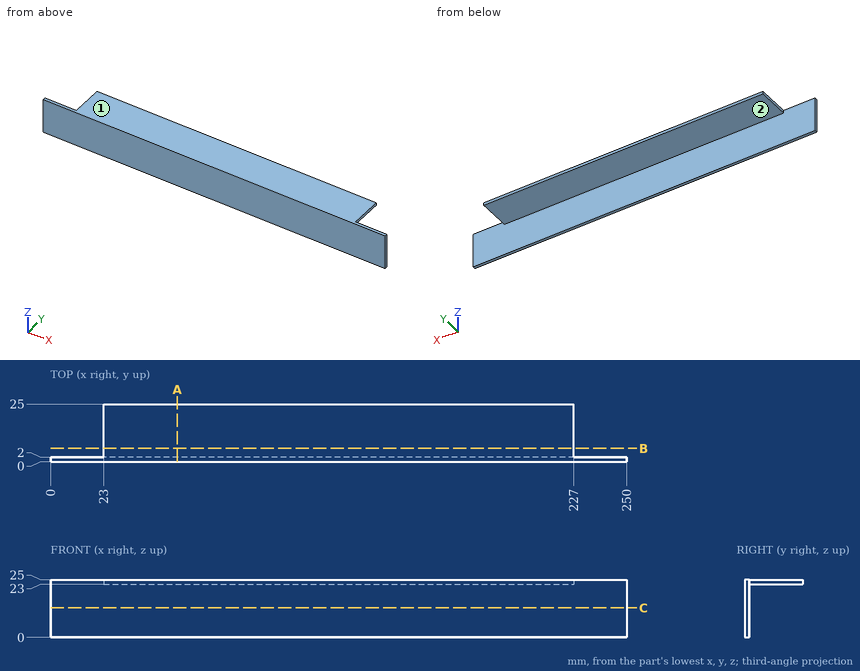
Input: dimensioned drawing with shaded views. Units: mm. Origin: part minimum x, y, z. A direction names the side the tool comes from. Coordinates: 2 decimals unless noted, no trailing zeros. Order: outer loops, then holes, each group sorted by start corner. A loop starts at its lowest first (then second) coordinate and runs counter-clockwise, first axis right, second up.
1. Ray query, line 1 along Y through (x, z) = (131.5, 4); line 2 along Z through (x, y) = (185, 15.5). Return the intervals inside material, ascending.
Checked values:
line 1: y = 0 to 2
line 2: z = 23 to 25
2. Cut plane C-C, the plane z = 12.75. Return loops of the section in (x, y).
Checked values:
outline: (0, 0) - (250, 0) - (250, 2) - (0, 2) - close
3. Access query for the marked faces 1 and 2. Directions: +Z, -Z, +X, -X, +Y, -Y. A direction counts if a zero-diameter tool reaches every point of the face in a straight line with its end or side. Return the directions, or none.
Checked values:
face 1: +Z, +X, -X, +Y, -Y
face 2: -Z, +X, -X, +Y
4. Contact query for flat-ended pins moving along their axis: P1, Ø12, axis at x = 221.5, y = 20.5, coming from the -Z side; P2, Ø12, axis at y = 12, z = 19, coming from the -X side; P3, Ø0.6, axis at y = 11.5, z = 24, coming from the +X side. Output: stop coordinate, or through.
Checked values:
P1: stops at z = 23
P2: stops at x = 23
P3: stops at x = 227
5. Cut plane A-A, the plane x = 55. Return loops of the section in (y, z).
Checked values:
outline: (0, 0) - (2, 0) - (2, 23) - (25, 23) - (25, 25) - (0, 25) - close
6. Cut plane B-B, the plane y = 5.75. Return loops of the section in (x, z), plus the area to 3 significant figures.
Checked values:
outline: (23, 23) - (227, 23) - (227, 25) - (23, 25) - close
area: 408 mm2
